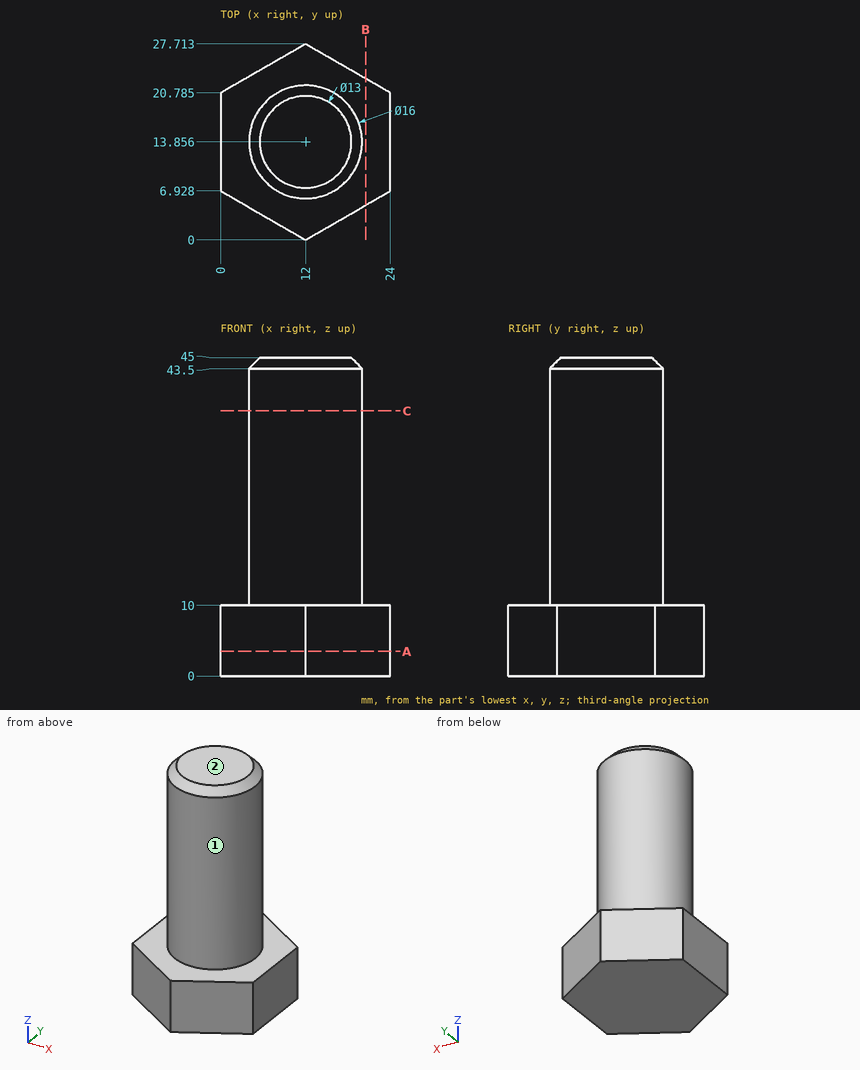
Can you work these out from the drawing? Everything is in mm from the part's minimum corner. A direction names the side the tool comes from. Give positions to 0.01 mm unless a question says otherwise; leave off trailing zeros. Loops run counter-clockwise (first coordinate to the right, second up) from the corner with the lowest first, then second, coordinate; pieces in that order, holes last. Notation, with made-up numbers: (58, 15) -> (115, 15) arc R10 ccw to (115, 19) -> close; hole circle Ø9 at (-2.75, -11.5). An arc over 180 degrees is marked (long way). Return JSON: item names as keys, results as strings.
Item 1: If we section it at C-C on z = 37.5: List the corners of the cut face in (x, y) for me.
Geometry results:
{"outline": "circle Ø16 at (12, 13.86)"}
Item 2: If we section it at A-A on z = 3.5: List the corners of the cut face in (x, y) for me (1 decimal), plus the area to 3 significant figures.
Geometry results:
{"outline": "(0, 6.9) -> (12, 0) -> (24, 6.9) -> (24, 20.8) -> (12, 27.7) -> (0, 20.8) -> close", "area": "499 mm²"}
Item 3: If we section it at B-B on x = 20.5: List the corners of the cut face in (y, z) for me (1 decimal), plus the area to 3 significant figures.
Geometry results:
{"outline": "(4.9, 0) -> (22.8, 0) -> (22.8, 10) -> (4.9, 10) -> close", "area": "179 mm²"}
Item 4: I need wall thicknesses on L1, parallel to Z at x = 7.75, y = 24; L2, parallel to Y at x = 12, z = 20; L3, parallel to X at y = 17, z = 28 (1 decimal). Which ranges of each line are inside material? Lowest first, please. Write a range as from..to.
Geometry results:
{"L1": "z = 0..10", "L2": "y = 5.86..21.86", "L3": "x = 4.6..19.4"}
Item 5: Which directions (+Z, -Z, +X, -X, +Y, -Y) give clear straight access to the entire face, cutting with the end or side of a thin tool? Please do the marked faces 1 and 2.
Geometry results:
{"face 1": "+Z", "face 2": "+Z, +X, -X, +Y, -Y"}
Item 6: I'm going to push flat-ended pins straight in: pin 1 (2 mm diameter, centred on y = 19, z = 13, fed in from -X); pin 2 (1 mm diameter, centred on x = 5, z = 13, fed in from +Y); pin 3 (6 mm diameter, centred on x = 20, z = 35, fed in from -Y). Where does each tip first touch, or does it pass through?
Geometry results:
{"pin 1": "stops at x = 5.16", "pin 2": "stops at y = 18.52", "pin 3": "stops at y = 7.61"}
